Check sheet for the drawn part. Datum: minimum x, y, z corner. Units: mm. A direction names the side the tool comes from. Round coordinates to 2 decimals unless told otherwise and drop trailing zeros. Order: outer loops, then holes, each group sorted by start corner. A loop starts at its lowest first (then second) coordinate and runs counter-clockwise, first axis right, second up. Notation, with made-up numbers: (24.5, 24) -> (49.5, 24) arc R32 cw to (49.5, 58) -> close; hole circle Ø8 at (48.25, 62.5). An arc over 180 degrees is marked (long way). Write item = value, one per line. Start each with the question number.
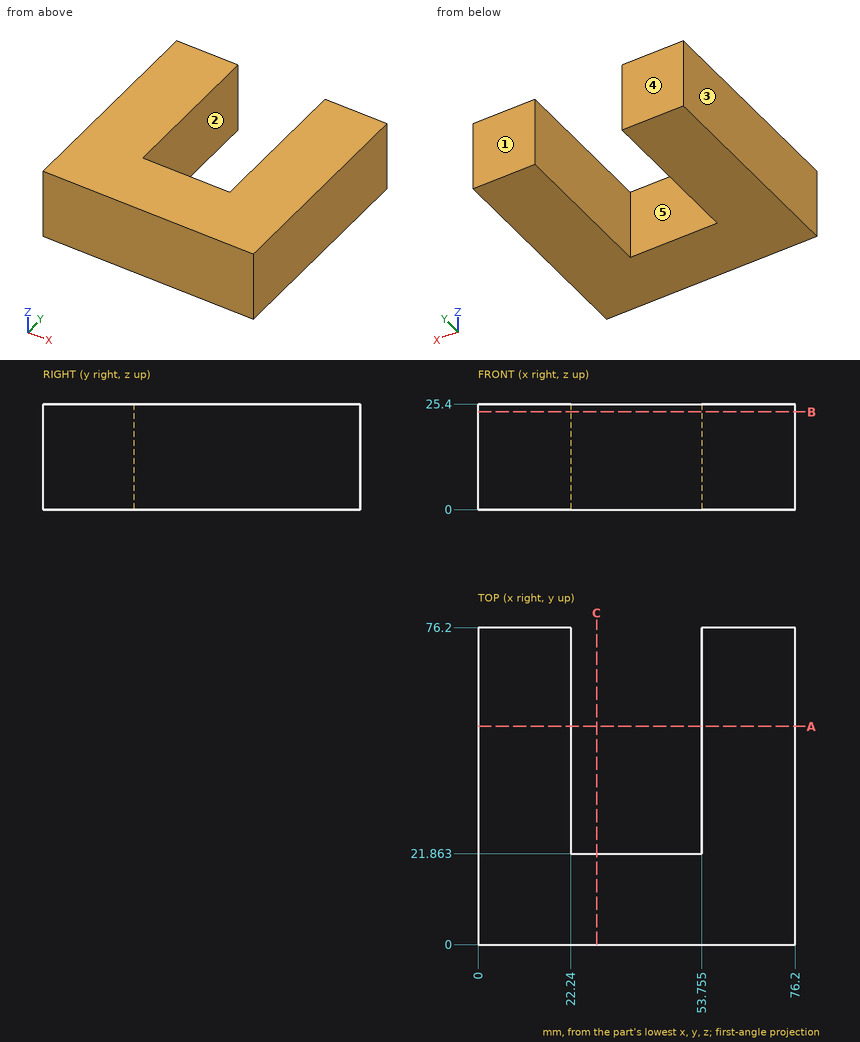
(1) Scan lines: line 1 along X through (y, z) = (72, 11.25) (1 decimal); line 2 along Y through (x, z) = (49.5, 3). Record each from-to range of solid material in increasing order. Write a range as from..to.
(2) Set-up check for the marked faces 1 and 2: record each of +Z, -Z, +X, -X, +Y, -Y from which the full face is reachable in a straight line by a thin tool's end or side.
(3) Depth check by flat-ended pin: pin 1 (1 mm diameter, centred on x = 52, z = 6.5, fed in from +Y). Enter the tip coordinate at first touch or a pass-through.
(4) Draft check along X on the marked faces 3, 4 and 5. Enter one of: +X half, -X half, draft (parallel to the pull), parting line (faces both ways), or undercut.
(5) Cross-section at C-C (x = 28.5). Enter the section's corners in (y, z), and give its area (3 significant figures).
(6) Cross-section at A-A (y = 52.5). Enter the section's corners in (x, z) (1 decimal).
(7) Cross-section at B-B (z = 23.5). Enter the section's corners in (x, y) (1 decimal), and give its area (3 significant figures).
Outcome:
q1.line_1 = 0..22.2, 53.8..76.2
q1.line_2 = 0..21.86
q2.face_1 = +Z, -Z, +X, -X, +Y
q2.face_2 = +Z, -Z, +Y
q3.pin_1 = 21.86
q4.face_3 = -X half
q4.face_4 = draft
q4.face_5 = undercut
q5.outline = (0, 0) -> (21.86, 0) -> (21.86, 25.4) -> (0, 25.4) -> close
q5.area = 555 mm^2
q6.outline = (0, 0) -> (22.2, 0) -> (22.2, 25.4) -> (0, 25.4) -> close; (53.8, 0) -> (76.2, 0) -> (76.2, 25.4) -> (53.8, 25.4) -> close
q7.outline = (0, 0) -> (76.2, 0) -> (76.2, 76.2) -> (53.8, 76.2) -> (53.8, 21.9) -> (22.2, 21.9) -> (22.2, 76.2) -> (0, 76.2) -> close
q7.area = 4,090 mm^2
